The model under review builds one solid part; all positions refer to its coordinate system, in mm. A direction names the side the tool comes from. Round coordinates to 2 decimals unless told otherwise and drop trailing zeros. Write each loop counter-clockwise with the first axis right and the second up, starting at its lowest first coordinate (ties: lowest second). Pieces come first, ordered by that corner, then holes. Notation, with made-up numbers: (9, 62.25) - (49, 62.25) arc R12 ccw to (49, 69.25) - close; hole circle Ø8 at (45, 18.25). An arc over 180 degrees is marked (long way). Return JSON: item names as keys, results as strings.
from build123d import *

# Parameters (mm, degrees)
F1_DEPTH = 25
F2_W     = 16.760172
F2_H     = 5
F3_DEPTH = 25


with BuildPart() as f1:
    # F0 (on Front) → F1 (new body)
    with BuildSketch(Plane.XZ):
        Polygon((21.915637, 3.063245), (-5.084363, 3.063245), (-5.084363, 0.063245), (23.915568, 0), (27.208995, 1.75), (32.208995, 1.75), (34.042088, 2.632186), (34.042088, 5.450061), (32.16216, 4.75), (25.09004, 4.75), align=None)
    extrude(amount=F1_DEPTH)

    # F2 (on face) → F3 (cut)
    with BuildSketch(Plane.XY.offset(3.063245)):
        with Locations((8.380086, -5.5)):
            Rectangle(F2_W, F2_H)
        with Locations((8.380086, -19.5)):
            Rectangle(F2_W, F2_H)
    extrude(amount=-F3_DEPTH, mode=Mode.SUBTRACT)


solid = f1.part
(1) Add section D-D (y = -2.25). Write out the cut boundary in (x, z), plus the area to 3 significant figures.
Filled in:
{"outline": "(-5.08, 0.06) - (23.92, 0) - (27.21, 1.75) - (32.21, 1.75) - (34.04, 2.63) - (34.04, 5.45) - (32.16, 4.75) - (25.09, 4.75) - (21.92, 3.06) - (-5.08, 3.06) - close", "area": "122 mm2"}
(2) Mouldability with a two-part tool opening along Y and no side actions: class faces 1 (the flat face through (14, -25, 2)), 2 (the flat face through (14, 0, 2)), 3 (the flat face through (8, -22, 2)), 4 (the flat face through (33.1, -12.3, 5.1)) as released by +Y, released by -Y, zero draft, split by the parting line, or undercut.
Filled in:
{"face 1": "released by -Y", "face 2": "released by +Y", "face 3": "undercut", "face 4": "zero draft"}
(3) Add section A-A (y = -6.5). Write out the cut boundary in (x, z), plus the area to 3 significant figures.
Filled in:
{"outline": "(-5.08, 0.06) - (0, 0.05) - (0, 3.06) - (-5.08, 3.06) - close; (16.76, 0.02) - (23.92, 0) - (27.21, 1.75) - (32.21, 1.75) - (34.04, 2.63) - (34.04, 5.45) - (32.16, 4.75) - (25.09, 4.75) - (21.92, 3.06) - (16.76, 3.06) - close", "area": "71.0 mm2"}
(4) Add section C-C (z = 0.9). Write out the cut boundary in (x, y).
Filled in:
{"outline": "(-5.08, -25) - (25.61, -25) - (25.61, 0) - (-5.08, 0) - close; hole (0, -22) - (16.76, -22) - (16.76, -17) - (0, -17) - close; hole (0, -8) - (16.76, -8) - (16.76, -3) - (0, -3) - close"}
(5) For faces 5 (the flat face through (9, -12, 3.063)), 6 (the flat face through (30, -12, 1.75)), 7 (the flat face through (8, -3, 2)), list the 3-axis set-ups (+Z, -Z, +X, -X, +Y, -Y) from which the entire face can be reached by the end or side of a thin tool; tool diameter is ignored.
Filled in:
{"face 5": "+Z, -X, +Y, -Y", "face 6": "-Z, +X, +Y, -Y", "face 7": "+Z, -Z"}
(6) Wall thickness on line 1 (Y direction, x = 14, z = 2.85); line 2 (Z direction, x = 1.5, y = -22.5); line 3 (Z direction, x = 29, y = -10): over which ranges is each line inside the solid? List them lowest first.
Filled in:
{"line 1": "y = -25 to -22, -17 to -8, -3 to 0", "line 2": "z = 0.05 to 3.06", "line 3": "z = 1.75 to 4.75"}
(7) Add section B-B (x = 7). Write out the cut boundary in (y, z).
Filled in:
{"outline": "(-25, 0.04) - (-22, 0.04) - (-22, 3.06) - (-25, 3.06) - close; (-17, 0.04) - (-8, 0.04) - (-8, 3.06) - (-17, 3.06) - close; (-3, 0.04) - (0, 0.04) - (0, 3.06) - (-3, 3.06) - close"}
(8) Clearance check with flat-ended pins moving along their axes: pin 1 Ø1.5 at (x, y) = (29.5, -8.5) entering from +Z; pin 2 Ø2 at (x, y) = (16, -22) entering from -Z; pin 3 Ø4 at (x, y) = (30, -7) entering from -Z. State where each tip first meets the part, or that it passes through.
Filled in:
{"pin 1": "stops at z = 4.75", "pin 2": "stops at z = 0.02", "pin 3": "stops at z = 1.75"}
